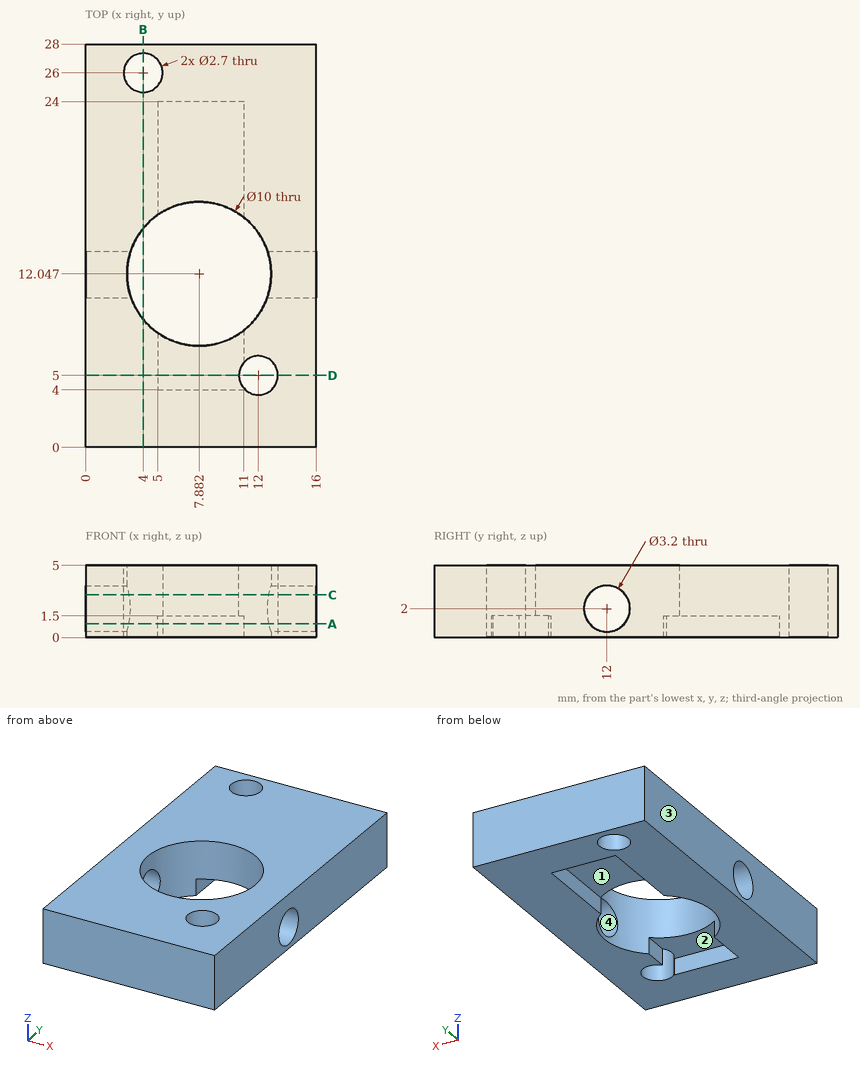
The figure shows three views and two pictorial views of one solid part (mm, origin at its lowest corner). Answer the questions. Give positions to 0.01 mm unless a question says otherwise; leave off trailing zeros. Order: outer loops, then holes, each group sorted by start corner. A loop starts at its lowest first (then second) coordinate and runs counter-clockwise, first axis right, second up. Notation, with made-up numbers: (-4.5, 43) -> (47.5, 43) arc R25 cw to (47.5, 80) -> close; hole circle Ø10 at (-31.75, 36.5). An arc over 180 degrees is marked (long way). Answer as CSV lines item,"result". Start each with the question number.
Q1. A cutting plane is placed at C-C (z = 2.95). Determine the outline of the cut face in (x, y), then the cut area to 3 significant figures.
Q2. A cutting plane is placed at D-D (y = 5). Determine the outline of the cut face in (x, z).
Q3. A cutting plane is placed at B-B (x = 4). Determine the outline of the cut face in (y, z), then the cut area to 3 significant figures.
Q4. A cutting plane is placed at A-A (z = 0.95). Determine the outline of the cut face in (x, y), then the cut area to 3 significant figures.
Q5. Given pin 1 (1.6 mm diameter, centred on x = 6.5, z = 0.5, fed in from -Y); pin 2 (1.6 mm diameter, centred on x = 4, y = 26, fed in from +Z); pin 3 (2 mm diameter, centred on x = 6.5, y = 8, fed in from -Z), each flat-ended and moving along its own axis, determine where each tip first touches the part or whether it passes through.
Q6. Find the intervals of material crossed by L1, parallel to Z at x = 14.2, y = 12; L2, parallel to Y at x = 11.25, z = 4.65; L3, parallel to Y at x = 3.5, z = 2.7 (1 decimal), in increasing order.
Q7. Determine the mould class of the marked faces 1, 2, 3 and 4 for opening direction X: pulls with the +X half, pulls with the -X half, needs draft (parallel to the pull), parting line crosses it, or undercut.
Results found:
1,outline,"(0, 0) -> (16, 0) -> (16, 10.71) -> (12.7, 10.71) arc R5 cw to (3.06, 10.71) -> (0, 10.71) -> close; (0, 13.29) -> (3.04, 13.29) arc R5 cw to (12.73, 13.29) -> (16, 13.29) -> (16, 28) -> (0, 28) -> close; hole circle Ø2.7 at (4, 26); hole circle Ø2.7 at (12, 5)"
1,area,"342 mm2"
2,outline,"(0, 0) -> (5, 0) -> (5, 1.5) -> (10.65, 1.5) -> (10.65, 5) -> (0, 5) -> close; (13.35, 0) -> (16, 0) -> (16, 5) -> (13.35, 5) -> close"
3,outline,"(0, 0) -> (8.9, 0) -> (8.9, 5) -> (0, 5) -> close; (15.2, 0) -> (24.65, 0) -> (24.65, 5) -> (15.2, 5) -> close; (27.35, 0) -> (28, 0) -> (28, 5) -> (27.35, 5) -> close"
3,area,"95.0 mm2"
4,outline,"(0, 0) -> (16, 0) -> (16, 10.79) -> (12.72, 10.79) arc R5 cw to (11, 8.14) -> (11, 5.91) arc R1.35 cw (long way) to (11, 4.09) -> (11, 4) -> (5, 4) -> (5, 7.96) arc R5 cw to (3.04, 10.79) -> (0, 10.79) -> close; (0, 13.21) -> (3.02, 13.21) arc R5 cw to (5, 16.13) -> (5, 24) -> (11, 24) -> (11, 15.96) arc R5 cw to (12.75, 13.21) -> (16, 13.21) -> (16, 28) -> (0, 28) -> close; hole circle Ø2.7 at (4, 26)"
4,area,"280 mm2"
5,pin 1,"y = 0"
5,pin 2,"through"
5,pin 3,"z = 1.5"
6,L1,"0 to 0.4, 3.6 to 5"
6,L2,"0 to 3.88, 6.12 to 8.35, 15.74 to 28"
6,L3,"0 to 9.6, 14.5 to 24.7, 27.3 to 28"
7,face 1,"undercut"
7,face 2,"undercut"
7,face 3,"pulls with the -X half"
7,face 4,"needs draft"
